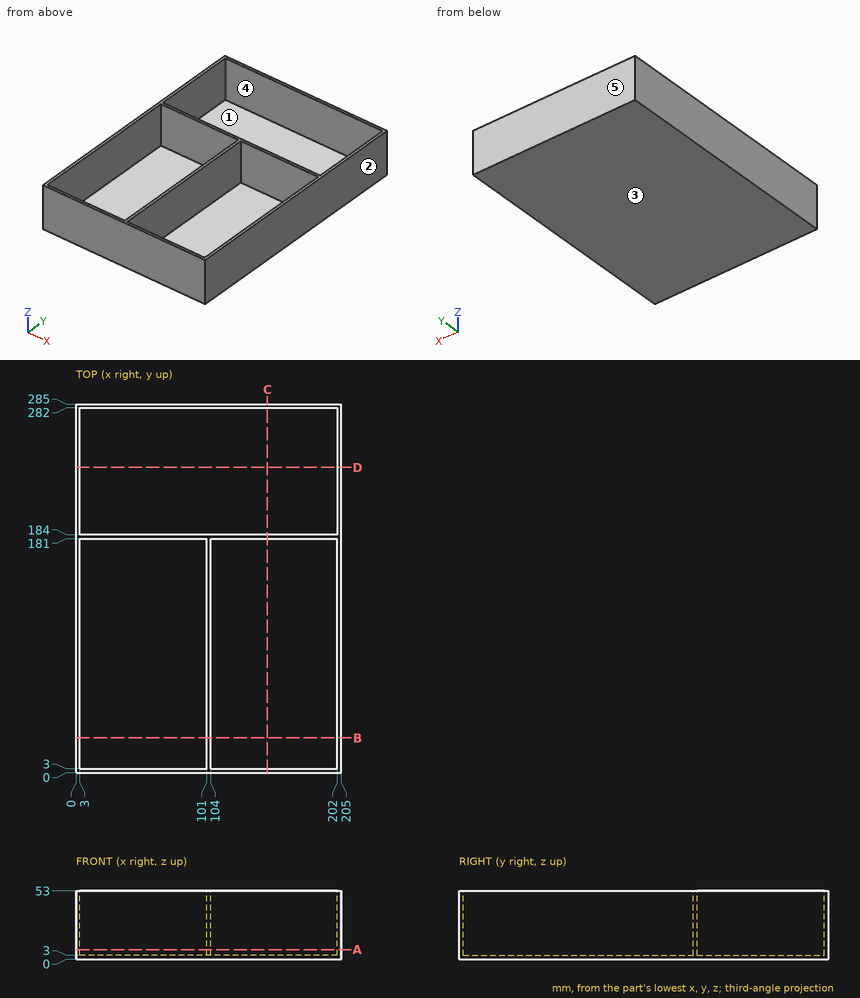
Study the drawing (mm; zero at the part's minimum x, y, z) and answer. A direction names the side the tool comes from. Give positions to 0.01 mm unless a question says otherwise; leave off trailing zeros. Loops run counter-clockwise (first coordinate to the right, second up) from the corner with the lowest first, then second, coordinate; pieces in that order, holes last. Notation, with made-up numbers: M 4,76.5 L 9,76.5 A18 cw 9,82.5 Z; hole C 78,47.5 d6. An arc over 180 degrees is marked long. One line per item, written item: value. Start each with the question number.
1. Which of the six approach directions +Z, -Z, +X, -X, +Y, -Y give full straight-line access (tool end or side, diameter ignored) to the marked faces 1 and 2?
2. Find section B-B (y = 27). Give the vertices of the cut face in (x, z).
3. This flat-tipped pin is pushed along its axis until it touches: P1, Ø1.5, axis at x = 100, y = 214.5, coming from the +Z side. Where does it stop, or does it pass through?
4. Find section D-D (y = 236). Give the vertices of the cut face in (x, z), and give its area (3 significant figures).
5. Find section A-A (z = 7.5). Give the vertices of the cut face in (x, y), and give its area (4 significant figures).
6. Determine the mould class of the marked faces 3, 4 and 5 for opening direction Y: released by +Y, released by -Y, zero draft, split by the parting line, or undercut.
7. Find the intervals of material crossed by probe 1 along Y at (x, z) = (125, 33.5); probe 2 along X at (y, z) = (92, 42); probe 3 along X at (y, z) = (237.5, 10), in increasing order.
8. Find section C-C (x = 148). Give the vertices of the cut face in (y, z).
Reported:
1. face 1: +Z
1. face 2: +Z, -Z, +X, +Y, -Y
2. outline: M 0,0 L 205,0 L 205,53 L 202,53 L 202,3 L 104,3 L 104,53 L 101,53 L 101,3 L 3,3 L 3,53 L 0,53 Z
3. P1: stops at z = 3
4. outline: M 0,0 L 205,0 L 205,53 L 202,53 L 202,3 L 3,3 L 3,53 L 0,53 Z
4. area: 915 mm²
5. outline: M 0,0 L 205,0 L 205,285 L 0,285 Z; hole M 3,3 L 101,3 L 101,181 L 3,181 Z; hole M 3,184 L 202,184 L 202,282 L 3,282 Z; hole M 104,3 L 202,3 L 202,181 L 104,181 Z
5. area: 4,035 mm²
6. face 3: zero draft
6. face 4: undercut
6. face 5: released by +Y
7. probe 1: y = 0 to 3, 181 to 184, 282 to 285
7. probe 2: x = 0 to 3, 101 to 104, 202 to 205
7. probe 3: x = 0 to 3, 202 to 205
8. outline: M 0,0 L 285,0 L 285,53 L 282,53 L 282,3 L 184,3 L 184,53 L 181,53 L 181,3 L 3,3 L 3,53 L 0,53 Z
